```python
from build123d import *

# Parameters (mm, degrees)
CUT_EXTRUDE1_DEPTH = 2


with BuildPart() as part:
    # Sketch1 → Revolve1 (revolve)
    with BuildSketch(Plane(origin=(0, 0, 0), x_dir=(0, 0, -1), z_dir=(1, 0, 0))):
        Polygon((0, -6), (1.5, -6), (1.5, 0), (2.85, 0), (2.85, 3), (0, 3), align=None)
    revolve(axis=Axis((0, 4, 0), (0, 1, 0)))

    # Sketch3 → Cut-Extrude1 (cut)
    with BuildSketch(Plane(origin=(0, 3, 0), x_dir=(1, 0, 0), z_dir=(0, 1, 0))):
        Polygon((1.443375673, 0), (0.721687836, 1.25), (-0.721687836, 1.25), (-1.443375673, 0), (-0.721687836, -1.25), (0.721687836, -1.25), align=None)
    extrude(amount=-CUT_EXTRUDE1_DEPTH, mode=Mode.SUBTRACT)


solid = part.part
```
Geometry check sheet. Reference: the model listing, model coordinates, mm. A direction names the side the tool comes from. Give positions to 0.01 mm unless a question says otherwise; leave off trailing zeros. Write each loop counter-clockwise with the first axis right and the second up, starting at its lowest first coordinate (ties: lowest second). Pieces come first, ordered by that corner, then holes.
1) Material ranges on L1, parallel to Y at x = -0.1, z = 2.2; L2, parallel to X at y = 2, z = -1.1; L3, parallel to Z at x = 0.55, y = -1, recorded low to high.
2) Access from +Z, -Z, +X, -X, +Y, -Y to the whole of each face (thin tool, end or side, straight path). Record for faces 4 (the flat face through (1.2, 0, 1.2)), 5 (the flat face through (0, 2, -1.25)), 6 (the cylindrical face through (1.734, 1.521, 2.262)).
3) Section check C-C, the plane y = -2.75. Record the boundary of the cut face in (x, z).
4) Gauge pin test, flat ends, axial feed: pin 1 (1.2 mm diameter, centred on x = -0.5, z = -0.5, fed in from +Y); pin 2 (1 mm diameter, centred on y = -3, z = -1, fed in from -X). Record the tip position at first contact, or that the pin passes through.
5) Release check for a two-part mould opening along Z. For faces 1 (the flat face through (-1.08, 2.01, -0.63)), 2 (the cylindrical face through (-0.07, -2.96, 1.5)), 3 (the flat face through (0, -6, 0)) record: pulls with the +Z half, pulls with the -Z half, needs draft (parallel to the pull), parting line crosses it, or undercut.
6) Section check A-A, the plane y = 1.5. Record the boundary of the cut face in (x, z).
7) Section check B-B, the plane x = 0. Record the boundary of the cut face in (y, z).
8) Section check D-D, the plane z = 2. Record the boundary of the cut face in (x, y), and give its area (3 significant figures).
Computed:
1. L1: y = 0 to 3
1. L2: x = -2.63 to -0.81, 0.81 to 2.63
1. L3: z = -1.4 to 1.4
2. face 4: -Y
2. face 5: +Y
2. face 6: +Y, -Y
3. outline: circle Ø3 at (0, 0)
4. pin 1: stops at y = 3
4. pin 2: stops at x = -1.41
5. face 1: undercut
5. face 2: parting line crosses it
5. face 3: needs draft
6. outline: circle Ø5.7 at (0, 0); hole (-1.44, 0) - (-0.72, -1.25) - (0.72, -1.25) - (1.44, 0) - (0.72, 1.25) - (-0.72, 1.25) - close
7. outline: (-6, -1.5) - (0, -1.5) - (0, -2.85) - (3, -2.85) - (3, -1.25) - (1, -1.25) - (1, 1.25) - (3, 1.25) - (3, 2.85) - (0, 2.85) - (0, 1.5) - (-6, 1.5) - close
8. outline: (-2.03, 0) - (2.03, 0) - (2.03, 3) - (-2.03, 3) - close
8. area: 12.2 mm2
